```python
from build123d import *

# Parameters (mm, degrees)
BASE_EXTRUDE_DEPTH = 1.5
SKETCH12_W         = 5.5
SKETCH12_H         = 4.5
CUT_EXTRUDE5_DEPTH = 66.448452999
CUT_EXTRUDE7_DEPTH = 66.448452999


with BuildPart() as part:
    # Sketch1 → Base-Extrude (new body)
    with BuildSketch(Plane.XY):
        with BuildLine():
            Line((-43.5, 47), (0, 47))
            Line((0, 47), (43.5, 47))
            ThreePointArc((43.5, 47), (44.560660172, 46.560660172), (45, 45.5))
            Line((45, 45.5), (45, -45.5))
            ThreePointArc((45, -45.5), (44.560660172, -46.560660172), (43.5, -47))
            Line((43.5, -47), (36.2, -47))
            ThreePointArc((36.2, -47), (36.058578644, -46.941421356), (36, -46.8))
            Line((36, -46.8), (36, -45.7))
            ThreePointArc((36, -45.7), (35.941421356, -45.558578644), (35.8, -45.5))
            Line((35.8, -45.5), (33.082842712, -45.5))
            ThreePointArc((33.082842712, -45.5), (33.006306026, -45.515224093), (32.941421356, -45.558578644))
            Line((32.941421356, -45.558578644), (31.5, -47))
            Line((31.5, -47), (-24.8, -47))
            ThreePointArc((-24.8, -47), (-24.941421356, -46.941421356), (-25, -46.8))
            Line((-25, -46.8), (-25, -45.7))
            ThreePointArc((-25, -45.7), (-25.058578644, -45.558578644), (-25.2, -45.5))
            Line((-25.2, -45.5), (-26.661796764, -45.5))
            Line((-26.661796764, -45.5), (-28, -47))
            Line((-28, -47), (-35.8, -47))
            ThreePointArc((-35.8, -47), (-35.941421356, -47.058578644), (-36, -47.2))
            Line((-36, -47.2), (-36, -47.3))
            ThreePointArc((-36, -47.3), (-36.058578644, -47.441421356), (-36.2, -47.5))
            Line((-36.2, -47.5), (-39, -47.5))
            Line((-39, -47.5), (-45, -41.5))
            Line((-45, -41.5), (-45, 45.5))
            ThreePointArc((-45, 45.5), (-44.560660172, 46.560660172), (-43.5, 47))
        make_face()
    extrude(amount=BASE_EXTRUDE_DEPTH)

    # Sketch12 → Cut-Extrude5 (cut, through all)
    with BuildSketch(Plane.XY.offset(1.5)):
        with Locations((40.249857546, 37.75)):
            Rectangle(SKETCH12_W, SKETCH12_H)
        with Locations((-40.249857546, 37.75)):
            Rectangle(SKETCH12_W, SKETCH12_H)
    extrude(amount=-CUT_EXTRUDE5_DEPTH, mode=Mode.SUBTRACT)

    # Sketch13 → Cut-Extrude7 (cut, through all)
    with BuildSketch(Plane.XY):
        with BuildLine():
            Line((-28, 38), (28, 38))
            ThreePointArc((28, 38), (29.414213562, 37.414213562), (30, 36))
            Line((30, 36), (30, 0))
            ThreePointArc((30, 0), (29.414213562, -1.414213562), (28, -2))
            Line((28, -2), (-28, -2))
            ThreePointArc((-28, -2), (-29.414213562, -1.414213562), (-30, 0))
            Line((-30, 0), (-30, 36))
            ThreePointArc((-30, 36), (-29.414213562, 37.414213562), (-28, 38))
        make_face()
    extrude(amount=CUT_EXTRUDE7_DEPTH, mode=Mode.SUBTRACT)


solid = part.part
```
Source: CAD feature listing. Evaluate the final solid. Frame: model axes, mm. A direction names the side the tool comes from. Round coordinates to 2 decimals unless told otherwise and drop trailing zeros. Write each loop counter-clockwise with the first axis right and the second up, starting at its lowest first coordinate (ties: lowest second). Pieces come first, ordered by that corner, then holes. Notation, with made-up numbers: M 50.25,71 L 77.25,71 A17 ccw 77.25,90 Z; hole C 81,-33.5 d10. An arc over 180 degrees is marked long. Answer as a JSON object with one key per item and string values. Group by question number.
(1) Section query C-C on z = 0.75. State how many separate pieces and enclosed holes the cut face has, then the cut area to 3 significant figures.
(2) Section query B-B on x = 0. Output: boundary loops of the cut face in (y, z), then the cut area to 3 significant figures.
(3) Reachability of faces 1 (the cylindrical face through (29.4, 37.43, 0.74)), 2 (the flat face through (1, -10, 1.5)) from +Z, -Z, +X, -X, +Y, -Y: full face, straight path, thin tool, end or side. Return the list, or none.
(4) First-contact query: pin 1 (0.5 mm diameter, centred on y = -46.5, z = 1, fed in from -X); pin 2 (0.8 mm diameter, centred on x = -7.5, z = 1, fed in from -Y); pin 3 (0.8 mm diameter, centred on x = 34, z = 0.5, fed in from -Y). Flat tips, straight axial feed; report the tip coordinate or a pass-through.
(5) Ray query, line 1 (X direction, y = 38.5, z = 1.05); line 2 (X direction, y = 10, z = 1.4); line 3 (Y direction, x = -17, z = 1.35). Return the intervals inside material, ascending. Write a range as [from, to].
(6) Mould query, pull axis X, two halves, no side actions, for faces 3 (the cylindrical face through (-29.4, -1.43, 0.74)), 4 (the flat face through (-42, -44.5, 0.7)), 5 (the flat face through (1, -10, 0)), 6 (the cylindrical face through (29.43, -1.4, 0.74)). Classes: +X half, -X half, draft (parallel to the pull), parting line (faces both ways), or undercut.
(7) Section query A-A on y = 12. Output: boundary loops of the cut face in (x, z), then the cut area to 3 significant figures.
Computed values:
{
 "1": {"separate pieces": "1", "enclosed holes": "3", "area": "5,990 mm^2"},
 "2": {"outline": "M -47,0 L -2,0 L -2,1.5 L -47,1.5 Z; M 38,0 L 47,0 L 47,1.5 L 38,1.5 Z", "area": "81.0 mm^2"},
 "3": {"face 1": "+Z, -Z", "face 2": "+Z, +X, -X, +Y, -Y"},
 "4": {"pin 1": "x = -40.25", "pin 2": "y = -47", "pin 3": "y = -45.5"},
 "5": {"line 1": "[-45, -43], [-37.5, 37.5], [43, 45]", "line 2": "[-45, -30], [30, 45]", "line 3": "[-47, -2], [38, 47]"},
 "6": {"face 3": "undercut", "face 4": "-X half", "face 5": "draft", "face 6": "undercut"},
 "7": {"outline": "M -45,0 L -30,0 L -30,1.5 L -45,1.5 Z; M 30,0 L 45,0 L 45,1.5 L 30,1.5 Z", "area": "45.0 mm^2"}
}
